```python
from build123d import *

# Parameters (mm, degrees)
F0_W     = 200
F0_H     = 100
F0_W_2   = 180
F0_H_2   = 80
F1_DEPTH = 50
F2_R     = 7.5
F3_DEPTH = 50


with BuildPart() as f1:
    # F0 (on Top) → F1 (new body)
    with BuildSketch(Plane.XY):
        Rectangle(F0_W, F0_H)
        Rectangle(F0_W_2, F0_H_2, mode=Mode.SUBTRACT)
    extrude(amount=F1_DEPTH)

    # F2 (on Front) → F3 (cut, symmetric)
    with BuildSketch(Plane.XZ):
        with Locations((0, 25)):
            Circle(F2_R)
        with Locations((-75, 25)):
            Circle(F2_R)
        with Locations((75, 25)):
            Circle(F2_R)
    extrude(amount=F3_DEPTH, both=True, mode=Mode.SUBTRACT)


solid = f1.part
```
Model file for the job. Use its own axes, mm. A direction names the side the tool comes from. Coordinates: 2 decimals unless noted, no trailing zeros. Order: outer loops, then holes, each group sorted by start corner. A loop starts at its lowest first (then second) coordinate and runs counter-clockwise, first axis right, second up. Notation, with made-up numbers: (72, 58.25) -> (107, 58.25) arc R5 ccw to (107, 62.25) -> close; hole circle Ø4 at (85.25, -10.75). An arc over 180 degrees is marked (long way). Answer as a JSON object with one key per item and string values. Group by question number.
1) Cut at B-B, the plane x = 0. Write the cut outline in (y, z).
2) Drill centre lines: L1, parallel to Z at x = 0, y = -44; L2, parallel to Y at x = 67.5, z = 45.5; L3, parallel to X at y = 2, z = 12. Where is each one in solid material? Low to high.
3) Which spindle directions (+Z, -Z, +X, -X, +Y, -Y) get a long thin tool onto all of the face, cutting with end or side? Do faces 5 (the face through (90, -1, 25)), 6 (the face through (100, -1, 25)). Say none if no direction does.
4) Cut at A-A, the plane z = 44. Write the cut outline in (x, y).
5) Pull direction X, two halves, no side cores. Call faces 1 (the face through (69.5, 44.9, 30.1)), 2 (the face through (-1, 50, 14)), 3 (the face through (-100, -1, 25)), 4 (the face through (-1, 40, 14)): +X half, -X half, draft (parallel to the pull), parting line (faces both ways), or undercut.
6) Flat gauge pin, fed straight in: pin 1 (13.5 mm diameter, centred on x = -75, z = 25, fed in from +Y). Where does the tip first touch, or does it go through?
7) Cut at D-D, the plane x = -36. Write the cut outline in (y, z), then the cut area to 3 significant figures.
8) Cut at C-C, the plane y = 29.5. Write the cut outline in (x, z).
Check values:
{
 "1": {"outline": "(-50, 0) -> (-40, 0) -> (-40, 17.5) -> (-50, 17.5) -> close; (-50, 32.5) -> (-40, 32.5) -> (-40, 50) -> (-50, 50) -> close; (40, 0) -> (50, 0) -> (50, 17.5) -> (40, 17.5) -> close; (40, 32.5) -> (50, 32.5) -> (50, 50) -> (40, 50) -> close"},
 "2": {"L1": "z = 0 to 17.5, 32.5 to 50", "L2": "y = -50 to -40, 40 to 50", "L3": "x = -100 to -90, 90 to 100"},
 "3": {"face 5": "+Z, -Z", "face 6": "+Z, -Z, +X, +Y, -Y"},
 "4": {"outline": "(-100, -50) -> (100, -50) -> (100, 50) -> (-100, 50) -> close; hole (-90, -40) -> (90, -40) -> (90, 40) -> (-90, 40) -> close"},
 "5": {"face 1": "undercut", "face 2": "draft", "face 3": "-X half", "face 4": "undercut"},
 "6": {"pin 1": "passes through"},
 "7": {"outline": "(-50, 0) -> (-40, 0) -> (-40, 50) -> (-50, 50) -> close; (40, 0) -> (50, 0) -> (50, 50) -> (40, 50) -> close", "area": "1,000 mm²"},
 "8": {"outline": "(-100, 0) -> (-90, 0) -> (-90, 50) -> (-100, 50) -> close; (90, 0) -> (100, 0) -> (100, 50) -> (90, 50) -> close"}
}
